Geometry: final body of the model. Coordinates: model frame, mm. Face numbers are marked on the shaded views. A direction names the side the tool comes from. Round coordinates to 2 decimals unless told otherwise and drop trailing zeros. Loops run counter-clockwise (first coordinate to the right, second up) from the corner with the lowest first, then second, coordinate; pieces in that order, holes last. Notation, with made-up numbers: M 47,46.25 L 82,46.25 A16 ccw 82,57.25 Z; hole C 56.25,67 d6. An arc over 180 degrees is marked long. Write each question's results on one line, items separated by ' | '.
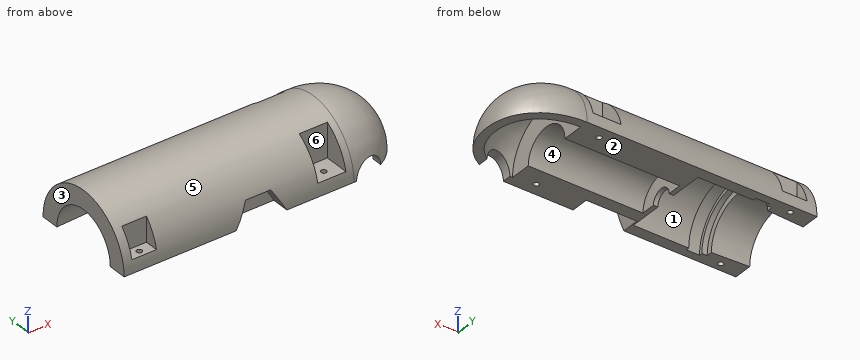
```python
from build123d import *

# Parameters (mm, degrees)
REVOLVE1_ANGLE          = 180
CUT_EXTRUDE1_REACH      = 114.566
CUT_EXTRUDE1_END_RADIUS = 31
SKETCH2_W               = 14
SKETCH2_H               = 8.465653043
SKETCH2_W_2             = 16
SKETCH2_H_2             = 15
CUT_EXTRUDE2_REACH      = 114.566
SKETCH3_R               = 1.525
CUT_EXTRUDE3_DEPTH      = 10
CUT_EXTRUDE4_REACH      = 128.25
SKETCH6_R               = 8.5


with BuildPart() as part:
    # Sketch1 → Revolve1 (revolve)
    with BuildSketch(Plane.XY):
        with BuildLine():
            Line((6.218316837, 14), (6.218316837, 6))
            Line((6.218316837, 6), (3.718316837, 6))
            Line((3.718316837, 6), (3.718316837, 24.731367941))
            Line((3.718316837, 24.731367941), (-10.171408573, 24.731367941))
            Line((-10.171408573, 24.731367941), (-27.781683163, 24.731367941))
            Line((-27.781683163, 24.731367941), (-27.781683163, 26.554502519))
            Line((-27.781683163, 26.554502519), (-35.281683163, 26.554502519))
            Line((-35.281683163, 26.554502519), (-35.281683163, 24.731367941))
            Line((-35.281683163, 24.731367941), (-38.281683163, 24.731367941))
            Line((-38.281683163, 24.731367941), (-38.281683163, 21.534346957))
            Line((-38.281683163, 21.534346957), (-59.281683163, 20.416426404))
            Line((-59.281683163, 20.416426404), (-59.281683163, 24.731367941))
            Line((-59.281683163, 24.731367941), (-59.281683163, 31))
            Line((-59.281683163, 31), (-56.981683163, 31))
            Line((-56.981683163, 31), (71.518316837, 31))
            add(Edge.make_bspline(
                [(71.518316837, 31), (87.336893309, 31), (105.518316837, 21.771712161), (105.518316837, 0)],
                knots=[0, 0, 0, 0, 1, 1, 1, 1], degree=3))
            Line((105.518316837, 0), (100.518316813, 0))
            add(Edge.make_bspline(
                [(71.518316837, 26), (84.501211561, 26), (100.518316813, 18.460024777), (100.518316813, 0)],
                knots=[0, 0, 0, 0, 1, 1, 1, 1], degree=3))
            Line((71.518316837, 26), (71.518316837, 14))
            Line((71.518316837, 14), (6.218316837, 14))
        make_face()
    revolve(axis=Axis((-52.937293729, 0, 0), (1, 0, 0)), revolution_arc=REVOLVE1_ANGLE)

    # Cut-Extrude1: up to this cylinder (the profile starts inside it)
    cut_extrude1_end = Plane(origin=(6.118317, 0, 0), z_dir=(-1, 0, 0)) * Cylinder(CUT_EXTRUDE1_END_RADIUS, 398.932, mode=Mode.PRIVATE)
    # Sketch2 → Cut-Extrude1 (cut, up to the surface)
    with BuildSketch(Plane(origin=(0, 0, 7), x_dir=(-1, 0, 0), z_dir=(0, 0, -1)), mode=Mode.PRIVATE) as cut_extrude1_sk1:
        with Locations((47.281683163, 26.767173479)):
            Rectangle(SKETCH2_W, SKETCH2_H)
    cut_extrude1_tool1 = extrude(cut_extrude1_sk1.sketch, amount=-CUT_EXTRUDE1_REACH, mode=Mode.PRIVATE) & cut_extrude1_end
    add(cut_extrude1_tool1.solids().sort_by_distance((-47.281683, 26.767173, 7))[0], mode=Mode.SUBTRACT)
    # Sketch2 → Cut-Extrude1 (cut, up to the surface)
    with BuildSketch(Plane(origin=(0, 0, 7), x_dir=(-1, 0, 0), z_dir=(0, 0, -1)), mode=Mode.PRIVATE) as cut_extrude1_sk2:
        with Locations((-59.518316837, -23.5)):
            Rectangle(SKETCH2_W_2, SKETCH2_H_2)
    cut_extrude1_tool2 = extrude(cut_extrude1_sk2.sketch, amount=-CUT_EXTRUDE1_REACH, mode=Mode.PRIVATE) & cut_extrude1_end
    add(cut_extrude1_tool2.solids().sort_by_distance((59.518317, -23.5, 7))[0], mode=Mode.SUBTRACT)
    # Sketch2 → Cut-Extrude1 (cut, up to the surface)
    with BuildSketch(Plane(origin=(0, 0, 7), x_dir=(-1, 0, 0), z_dir=(0, 0, -1)), mode=Mode.PRIVATE) as cut_extrude1_sk3:
        with Locations((-59.518316837, 23.5)):
            Rectangle(SKETCH2_W_2, SKETCH2_H_2)
    cut_extrude1_tool3 = extrude(cut_extrude1_sk3.sketch, amount=-CUT_EXTRUDE1_REACH, mode=Mode.PRIVATE) & cut_extrude1_end
    add(cut_extrude1_tool3.solids().sort_by_distance((59.518317, 23.5, 7))[0], mode=Mode.SUBTRACT)
    # Sketch2 → Cut-Extrude1 (cut, up to the surface)
    with BuildSketch(Plane(origin=(0, 0, 7), x_dir=(-1, 0, 0), z_dir=(0, 0, -1)), mode=Mode.PRIVATE) as cut_extrude1_sk4:
        with Locations((47.281683163, -26.767173479)):
            Rectangle(SKETCH2_W, SKETCH2_H)
    cut_extrude1_tool4 = extrude(cut_extrude1_sk4.sketch, amount=-CUT_EXTRUDE1_REACH, mode=Mode.PRIVATE) & cut_extrude1_end
    add(cut_extrude1_tool4.solids().sort_by_distance((-47.281683, -26.767173, 7))[0], mode=Mode.SUBTRACT)

    # Sketch3 → Cut-Extrude2 (cut, up to next)
    with BuildSketch(Plane.XY.offset(7), mode=Mode.PRIVATE) as cut_extrude2_sk1:
        with Locations((-47.281683163, 26.534346957)):
            Circle(SKETCH3_R)
    cut_extrude2_tool1 = extrude(cut_extrude2_sk1.sketch, amount=-CUT_EXTRUDE2_REACH, mode=Mode.PRIVATE) & part.part
    # Sketch3 → Cut-Extrude2 (cut, up to next)
    with BuildSketch(Plane.XY.offset(7), mode=Mode.PRIVATE) as cut_extrude2_sk2:
        with Locations(Location((-47.281683163, -26.534346957, 0), (0, 0, 90))):
            Circle(SKETCH3_R)
    cut_extrude2_tool2 = extrude(cut_extrude2_sk2.sketch, amount=-CUT_EXTRUDE2_REACH, mode=Mode.PRIVATE) & part.part
    # Sketch3 → Cut-Extrude2 (cut, up to next)
    with BuildSketch(Plane.XY.offset(7), mode=Mode.PRIVATE) as cut_extrude2_sk3:
        with Locations((59.518316837, 24)):
            Circle(SKETCH3_R)
    cut_extrude2_tool3 = extrude(cut_extrude2_sk3.sketch, amount=-CUT_EXTRUDE2_REACH, mode=Mode.PRIVATE) & part.part
    # Sketch3 → Cut-Extrude2 (cut, up to next)
    with BuildSketch(Plane.XY.offset(7), mode=Mode.PRIVATE) as cut_extrude2_sk4:
        with Locations((59.518316837, -24)):
            Circle(SKETCH3_R)
    cut_extrude2_tool4 = extrude(cut_extrude2_sk4.sketch, amount=-CUT_EXTRUDE2_REACH, mode=Mode.PRIVATE) & part.part
    add(cut_extrude2_tool1.solids().sort_by_distance((-47.281683, 26.534347, 7))[0], mode=Mode.SUBTRACT)
    add(cut_extrude2_tool2.solids().sort_by_distance((-47.281683, -26.534347, 7))[0], mode=Mode.SUBTRACT)
    add(cut_extrude2_tool3.solids().sort_by_distance((59.518317, 24, 7))[0], mode=Mode.SUBTRACT)
    add(cut_extrude2_tool4.solids().sort_by_distance((59.518317, -24, 7))[0], mode=Mode.SUBTRACT)

    # Sketch5 → Cut-Extrude3 (cut)
    with BuildSketch(Plane(origin=(0, -31, 0), x_dir=(1, 0, 0), z_dir=(0, 1, 0))):
        Polygon((4.441941487, 0), (11.658819852, -12.5), (26.092576582, -12.5), (33.309454947, 0), (26.092576582, 12.5), (11.658819852, 12.5), align=None)
    extrude(amount=CUT_EXTRUDE3_DEPTH, mode=Mode.SUBTRACT)

    # Sketch6 → Cut-Extrude4 (cut, up to next)
    with BuildSketch(Plane(origin=(0, -31, 0), x_dir=(1, 0, 0), z_dir=(0, 1, 0)), mode=Mode.PRIVATE) as cut_extrude4_sk1:
        with Locations((81.518316837, 0)):
            Circle(SKETCH6_R)
    cut_extrude4_tool1 = extrude(cut_extrude4_sk1.sketch, amount=CUT_EXTRUDE4_REACH, mode=Mode.PRIVATE) & part.part
    add(cut_extrude4_tool1.solids().sort_by_distance((81.518317, -31, 0))[0], mode=Mode.SUBTRACT)


solid = part.part
```
1. Ray query, probe 1 along X at (y, z) = (-27.5, 5); probe 2 along X at (y, z) = (-27, 2); probe 3 along X at (y, z) = (21.5, 10). Return the intervals inside material, ascending.
Answer key:
probe 1: x = -59.28 to -48.46, -46.1 to 7.33, 30.42 to 74.64 | probe 2: x = -59.28 to -48.73, -45.83 to 5.6, 32.15 to 73.26 | probe 3: x = -59.28 to -38.28, 3.72 to 51.52, 67.52 to 71.52, 83.94 to 94.39
2. Section A-A (x = -2.5). Output: boundary loops of the cut face in (y, z).
Answer key:
outline: M -31,0 L -24.73,0 A24.73 cw 24.73,0 L 31,0 A31 ccw Z
3. Access query for the marked faces 4, 5 and 6. Directions: +Z, -Z, +X, -X, +Y, -Y. A direction counts if a zero-diameter tool reaches every point of the face in a straight line with its end or side. Return the directions, or none.
Answer key:
face 4: -Z | face 5: +Z, +X, -X | face 6: +Z, -Y
4. Draft query along X for the marked faces 1, 2 and 3. Return one class per face: pulls with the +X half, pulls with the -X half, needs draft (parallel to the pull), parting line crosses it, or undercut.
Answer key:
face 1: undercut | face 2: needs draft | face 3: pulls with the -X half
5. Pin query (flat end, axial travel): P1, Ø12, axis at y = 13.5, z = 26, coming from the +X side; P2, Ø7, axis at y = 23.5, z = 20, coming from the +X side; P3, Ø4.5, axis at x = 58, y = -22.5, coming from the +Z side; P4, Ø2.5, axis at x = 59.52, y = 24, coming from the +Z side. Return the tip coordinate at first contact, or that it passes through.
Answer key:
P1: stops at x = 94.92 | P2: stops at x = 88.35 | P3: stops at z = 7 | P4: passes through
